The model under review builds one solid part; all positions refer to its coordinate system, in mm. Face numbers are marked on the shaded views. A direction names the side the tool comes from. Round coordinates to 2 decimals unless told otherwise and drop trailing zeros. Write each loop counter-clockwise with the first axis right and the second up, starting at its lowest first coordinate (ties: lowest second). Pieces come first, ordered by that corner, then holes. Notation, with made-up numbers: (53.25, -1.75) - (84.25, -1.75) arc R29 cw to (84.25, 34.25) - close; hole circle Ø3 at (69, -23). An arc over 180 degrees is marked (long way). Return JSON: item names as keys, results as strings.
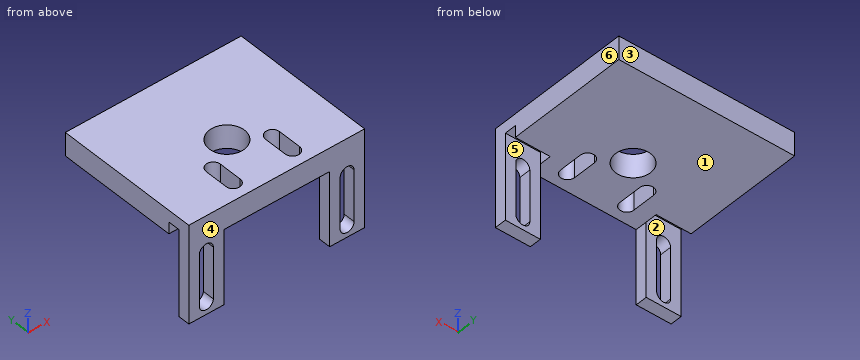
from build123d import *

# Parameters (mm, degrees)
SKETCH1_W           = 75.4
SKETCH1_H           = 62
SKETCH1_R           = 7.5
BOSS_EXTRUDE1_DEPTH = 10
SKETCH2_W           = 15
SKETCH2_H           = 32
BOSS_EXTRUDE2_DEPTH = 5
SKETCH3_W           = 15
SKETCH3_H           = 5
CUT_EXTRUDE1_DEPTH  = 5


with BuildPart() as part:
    # Sketch1 → Boss-Extrude1 (new body)
    with BuildSketch(Plane.XY):
        with Locations((0, 31)):
            Rectangle(SKETCH1_W, SKETCH1_H)
        with Locations((0, 25)):
            Circle(SKETCH1_R, mode=Mode.SUBTRACT)
        with BuildLine():
            Line((-9.7, 17), (-9.7, 7))
            ThreePointArc((-9.7, 7), (-12.7, 4), (-15.7, 7))
            Line((-15.7, 7), (-15.7, 17))
            ThreePointArc((-15.7, 17), (-12.7, 20), (-9.7, 17))
        make_face(mode=Mode.SUBTRACT)
        with BuildLine():
            Line((9.7, 17), (9.7, 7))
            ThreePointArc((9.7, 7), (12.7, 4), (15.7, 7))
            Line((15.7, 7), (15.7, 17))
            ThreePointArc((15.7, 17), (12.7, 20), (9.7, 17))
        make_face(mode=Mode.SUBTRACT)
    extrude(amount=BOSS_EXTRUDE1_DEPTH)

    # Sketch2 → Boss-Extrude2 (add)
    # profile 1 of 2: a face of its own
    with BuildSketch(Plane(origin=(0, 0, 0), x_dir=(1, 0, 0), z_dir=(0, 1, 0))):
        with Locations((-30.2, 16)):
            Rectangle(SKETCH2_W, SKETCH2_H)
        with BuildLine():
            Line((-27.2, 27), (-27.2, 5))
            ThreePointArc((-27.2, 5), (-30.2, 2), (-33.2, 5))
            Line((-33.2, 5), (-33.2, 27))
            ThreePointArc((-33.2, 27), (-30.2, 30), (-27.2, 27))
        make_face(mode=Mode.SUBTRACT)
    # profile 2 of 2: a face of its own
    with BuildSketch(Plane(origin=(0, 0, 0), x_dir=(1, 0, 0), z_dir=(0, 1, 0))):
        with Locations((30.2, 16)):
            Rectangle(SKETCH2_W, SKETCH2_H)
        with BuildLine():
            Line((27.2, 27), (27.2, 5))
            ThreePointArc((27.2, 5), (30.2, 2), (33.2, 5))
            Line((33.2, 5), (33.2, 27))
            ThreePointArc((33.2, 27), (30.2, 30), (27.2, 27))
        make_face(mode=Mode.SUBTRACT)
    extrude(amount=BOSS_EXTRUDE2_DEPTH)

    # Sketch3 → Cut-Extrude1 (cut)
    with BuildSketch(Plane.XY):
        with Locations((-30.2, 7.5)):
            Rectangle(SKETCH3_W, SKETCH3_H)
        with Locations((30.2, 7.5)):
            Rectangle(SKETCH3_W, SKETCH3_H)
    extrude(amount=CUT_EXTRUDE1_DEPTH, mode=Mode.SUBTRACT)


solid = part.part
(1) Mouldability with a two-part tool opening along Y and no side actions: class the marked faces 1, 2, 3 and 4 as released by +Y, released by -Y, zero draft, split by the parting line, or undercut.
Filled in:
{"face 1": "zero draft", "face 2": "undercut", "face 3": "released by +Y", "face 4": "released by -Y"}
(2) Add section D-D (y = 18.5). Write out the cut boundary in (x, z), plus the area to 3 significant figures.
Filled in:
{"outline": "(-37.7, 0) - (-15.3, 0) - (-15.3, 10) - (-37.7, 10) - close; (-10.1, 0) - (-3.74, 0) - (-3.74, 10) - (-10.1, 10) - close; (3.74, 0) - (10.1, 0) - (10.1, 10) - (3.74, 10) - close; (15.3, 0) - (37.7, 0) - (37.7, 10) - (15.3, 10) - close", "area": "575 mm2"}
(3) Add section B-B (x = 30.2). Write out the cut boundary in (y, z).
Filled in:
{"outline": "(0, -32) - (5, -32) - (5, -30) - (0, -30) - close; (0, -2) - (5, -2) - (5, 5) - (10, 5) - (10, 0) - (62, 0) - (62, 10) - (0, 10) - close"}
(4) For the marked faces 5 and 6, list the 3-axis set-ups (+Z, -Z, +X, -X, +Y, -Y) from which the entire face can be reached by the end or side of a thin tool; tool diameter is ignored.
Filled in:
{"face 5": "-Z, +X", "face 6": "+Z, -Z, +X, +Y, -Y"}
(5) Add section C-C (y = 12). Write out the cut boundary in (x, z).
Filled in:
{"outline": "(-37.7, 0) - (-15.7, 0) - (-15.7, 10) - (-37.7, 10) - close; (-9.7, 0) - (9.7, 0) - (9.7, 10) - (-9.7, 10) - close; (15.7, 0) - (37.7, 0) - (37.7, 10) - (15.7, 10) - close"}
(6) Add section A-A (z = -12). Write out the cut boundary in (x, y).
Filled in:
{"outline": "(-37.7, 0) - (-33.2, 0) - (-33.2, 5) - (-37.7, 5) - close; (-27.2, 0) - (-22.7, 0) - (-22.7, 5) - (-27.2, 5) - close; (22.7, 0) - (27.2, 0) - (27.2, 5) - (22.7, 5) - close; (33.2, 0) - (37.7, 0) - (37.7, 5) - (33.2, 5) - close"}
(7) Wall thickness on line 1 (X direction, y = 8.5, z = 4.5); line 2 (X direction, y = 4, z = -9.5); line 3 (X direction, y = 10.5, z = 2.5): over which ranges is each line inside the solid? List them lowest first.
Filled in:
{"line 1": "x = -22.7 to -15.7, -9.7 to 9.7, 15.7 to 22.7", "line 2": "x = -37.7 to -33.2, -27.2 to -22.7, 22.7 to 27.2, 33.2 to 37.7", "line 3": "x = -37.7 to -15.7, -9.7 to 9.7, 15.7 to 37.7"}
(8) Clearance check with flat-ended pins moving along their axes: pin 1 Ø2.5 at (x, y) = (32, 6.5) entering from -Z; pin 2 Ø12 at (x, z) = (-32.5, -17.5) entering from +Y. State where each tip first meets the part, or that it passes through.
Filled in:
{"pin 1": "stops at z = 5", "pin 2": "stops at y = 5"}
